Check sheet for the modelled part. Datum: model origin and axes. Units: mm. Coordinates: 2 decimals unless noted, no trailing zeros. Loops run counter-clockwise (first coordinate to the right, second up) from the corner with the lowest first, then second, coordinate; pieces in that order, holes last. Notation, with made-up numbers: M -26.75,6 L -12.75,6 A15 cw -12.75,10 Z; hole C -20.75,70.5 d9. An arc over 180 degrees is marked long. Return JSON: item names as keys, results as strings.
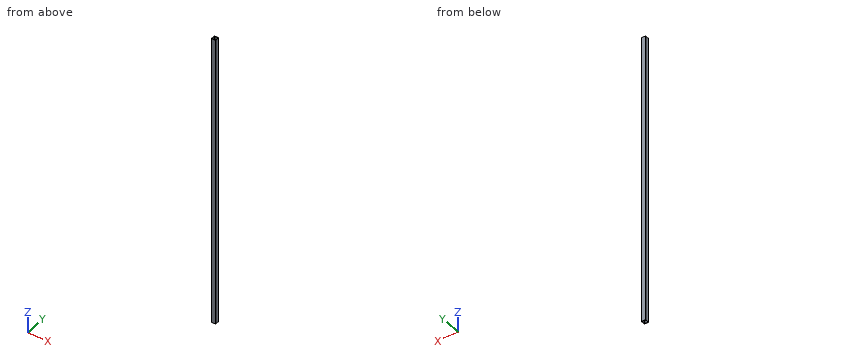
from build123d import *

# Parameters (mm, degrees)
SKETCH1_W           = 7.9
SKETCH1_H           = 7.9
SKETCH1_W_2         = 6.3
SKETCH1_H_2         = 6.3
BOSS_EXTRUDE1_DEPTH = 275
FILLET1_R           = 0.5


with BuildPart() as part:
    # Sketch1 → Boss-Extrude1 (new body, symmetric)
    with BuildSketch(Plane.XY):
        Rectangle(SKETCH1_W, SKETCH1_H)
        Rectangle(SKETCH1_W_2, SKETCH1_H_2, mode=Mode.SUBTRACT)
    extrude(amount=BOSS_EXTRUDE1_DEPTH, both=True)

    # Fillet1
    fillet1_edges = [part.edges().sort_by_distance(p)[0] for p in [
        (3.15, -3.15, 0),
        (3.15, 3.15, 0),
        (-3.15, 3.15, 0),
        (-3.15, -3.15, 0),
        (3.95, -3.95, 0),
        (-3.95, -3.95, 0),
        (-3.95, 3.95, 0),
        (3.95, 3.95, 0),
    ]]
    fillet(fillet1_edges, radius=FILLET1_R)


solid = part.part
1) Section check A-A on x = 1. Record the cut outline in (y, z).
Answers:
{"outline": "M -3.95,-275 L -3.15,-275 L -3.15,275 L -3.95,275 Z; M 3.15,-275 L 3.95,-275 L 3.95,275 L 3.15,275 Z"}
2) Section check C-C on z = -31. Record the cut outline in (x, y), then the cut area to 3 significant figures.
Answers:
{"outline": "M -3.95,-3.45 A0.5 ccw -3.45,-3.95 L 3.45,-3.95 A0.5 ccw 3.95,-3.45 L 3.95,3.45 A0.5 ccw 3.45,3.95 L -3.45,3.95 A0.5 ccw -3.95,3.45 Z; hole M -3.15,-2.65 A0.5 ccw -2.65,-3.15 L 2.65,-3.15 A0.5 ccw 3.15,-2.65 L 3.15,2.65 A0.5 ccw 2.65,3.15 L -2.65,3.15 A0.5 ccw -3.15,2.65 Z", "area": "22.7 mm²"}
3) Scan lines: line 1 along X through (y, z) = (2.75, 122); line 2 along Y through (x, z) = (2.5, -130). Record each from-to range of solid material in increasing order. Write a range as [from, to].
Answers:
{"line 1": "[-3.95, -3.14], [3.14, 3.95]", "line 2": "[-3.95, -3.15], [3.15, 3.95]"}
